Design review of the part built by this model. Coordinates are the model's own, in mm. Face numbers are marked on the shaded views. A direction names the side the tool comes from. Coordinates: 2 decimals unless noted, no trailing zeros. Write each loop counter-clockwise with the first axis right and the second up, starting at its lowest first coordinate (ties: lowest second). Pieces come first, ordered by that corner, then holes.
Q1. Add section D-D, the plane y = -10.5. Give the boundary of the cut face in (x, z), plus the area to 3 significant figures.
Q2. Add section C-C, the plane x = 11.5. Give the boundary of the cut face in (y, z).
Q3. Clearance check with flat-ended pins moving along their axes: pin 1 Ø2 at (x, z) = (-7.5, -6.5) entering from +Y; pin 2 Ø8 at (x, y) = (1, -2.5) entering from -Z; pin 3 Ø1 at (y, z) = (7, -5.5) entering from +X; pin 4 Ø6 at (x, y) = (0, 0) entering from -Z. State where each tip first meets the part, or that it passes through.
Q4. Machinability: for the marked faces 1, 2 and 3, which of the approach directions +Z, -Z, +X, -X, +Y, -Y give a long, thin tool a straight path to every point of the face, cutting with its end or side? Answer none if there is none.
Q5. The part is to be moulded in two halves that separate along Y. For the marked faces 4, 5 and 6, say which applies: +Y half, -Y half, draft (parallel to the pull), parting line (faces both ways), or undercut.
Q6. Add section A-A, the plane y = 0. Give the boundary of the cut face in (x, z), plus the area to 3 significant figures.
Q7. To check wall thickness, follow probe 1 along X at (y, z) = (0.25, -5.25); probe 2 along Y at (x, z) = (0, 0.5). State the ranges of each line that lie inside material, in increasing order.
from build123d import *

# Parameters (mm, degrees)
SKETCH013_R           = 14.5
PAD005_DEPTH          = 8.4
PAD006_DEPTH          = 0.9
POLARPATTERN006_COUNT = 8
SKETCH023_R           = 12.5
POCKET008_DEPTH       = 5
SKETCH017_R           = 5.25
POCKET006_DEPTH       = 1.4
SKETCH018_R           = 3.2
POCKET007_DEPTH       = 8.401
POCKET007_DEPTH_BACK  = 0.901


with BuildPart() as part:
    # Sketch013 → Pad005 (new body)
    with BuildSketch(Plane.XY):
        Circle(SKETCH013_R)
    extrude(amount=-PAD005_DEPTH)

    # Sketch016 → Pad006 (join)
    with BuildSketch(Plane.XY):
        with BuildLine():
            ThreePointArc((0.9499750638, 6.9568831834), (0, 7.9), (-0.9499750638, 6.9568831834))
            Line((-0.9499750638, 6.9568831834), (-0.9566171674, 6.0401804808))
            ThreePointArc((-1.9134171618, 4.6193976626), (-1.2209267144, 5.1856138051), (-0.9566171674, 6.0401804808))
            Line((-1.9134171618, 4.6193976626), (0, 0))
            Line((0, 0), (1.9134171618, 4.6193976626))
            ThreePointArc((0.9566171674, 6.0401804808), (1.2209267144, 5.1856138051), (1.9134171618, 4.6193976626))
            Line((0.9499750638, 6.9568831834), (0.9566171674, 6.0401804808))
        make_face()
    pad006 = extrude(amount=PAD006_DEPTH)

    # PolarPattern006: Pad006 ×8 about axis
    polarpattern006_axis = Axis((0, 0, 0), (0, 0, 1))
    for i in range(1, POLARPATTERN006_COUNT):
        add(pad006.rotate(polarpattern006_axis, i * 360 / POLARPATTERN006_COUNT))

    # Sketch023 → Pocket008 (cut)
    with BuildSketch(Plane.XY.offset(-8.4)):
        Circle(SKETCH023_R)
    extrude(amount=POCKET008_DEPTH, mode=Mode.SUBTRACT)

    # Sketch017 → Pocket006 (cut)
    with BuildSketch(Plane.XY.offset(-3.4)):
        Circle(SKETCH017_R)
    extrude(amount=POCKET006_DEPTH, mode=Mode.SUBTRACT)

    # Sketch018 → Pocket007 (cut, two sides)
    with BuildSketch(Plane.XY) as pocket007_sk:
        Circle(SKETCH018_R)
    extrude(amount=-POCKET007_DEPTH, mode=Mode.SUBTRACT)
    extrude(pocket007_sk.sketch, amount=POCKET007_DEPTH_BACK, mode=Mode.SUBTRACT)


solid = part.part
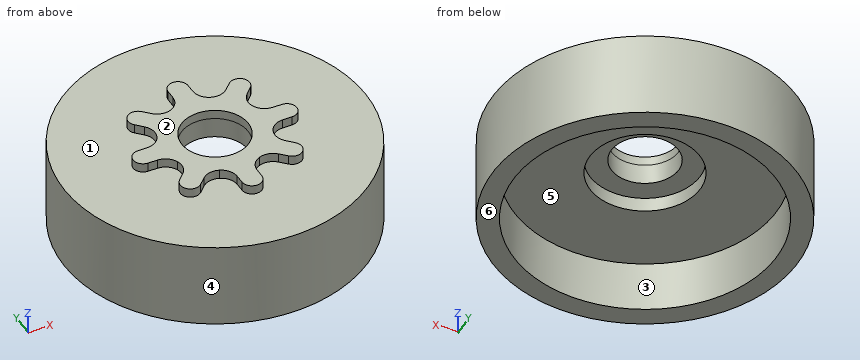
Here are the results:
1. outline: (-10, -8.4) - (-6.78, -8.4) - (-6.78, -3.4) - (6.78, -3.4) - (6.78, -8.4) - (10, -8.4) - (10, 0) - (-10, 0) - close
1. area: 100 mm2
2. outline: (-8.83, -8.4) - (-4.9, -8.4) - (-4.9, -3.4) - (4.9, -3.4) - (4.9, -8.4) - (8.83, -8.4) - (8.83, 0) - (-8.83, 0) - close
3. pin 1: stops at y = 12.96
3. pin 2: stops at z = -3.4
3. pin 3: stops at x = 12.96
3. pin 4: passes through
4. face 1: +Z
4. face 2: +Z, +X, -X, +Y, -Y
4. face 3: -Z
5. face 4: parting line
5. face 5: undercut
5. face 6: draft
6. outline: (-14.5, -8.4) - (-12.5, -8.4) - (-12.5, -3.4) - (-5.25, -3.4) - (-5.25, -2) - (-3.2, -2) - (-3.2, 0.9) - (-7.9, 0.9) - (-7.9, 0) - (-14.5, 0) - close; (3.2, -2) - (5.25, -2) - (5.25, -3.4) - (12.5, -3.4) - (12.5, -8.4) - (14.5, -8.4) - (14.5, 0) - (7.9, 0) - (7.9, 0.9) - (3.2, 0.9) - close
6. area: 99.6 mm2
7. probe 1: x = -14.5 to -12.5, 12.5 to 14.5
7. probe 2: y = -7.9 to -3.2, 3.2 to 7.9
